from build123d import *

# Parameters (mm, degrees)
SKETCH1_R           = 12.7
BOSS_EXTRUDE1_DEPTH = 7.9248
SKETCH2_R           = 9.525
BOSS_EXTRUDE2_DEPTH = 13.2715
SKETCH3_R           = 5.6388
BOSS_EXTRUDE3_DEPTH = 9.525
BOSS_EXTRUDE4_START = 6.35
SKETCH4_R           = 9.525
BOSS_EXTRUDE4_DEPTH = 6.35
SKETCH5_R           = 8.636
BOSS_EXTRUDE5_DEPTH = 9.525
SKETCH6_R           = 6.35
CUT_EXTRUDE1_DEPTH  = 25.4
SKETCH7_R           = 3.175
CUT_EXTRUDE2_DEPTH  = 32.108519733


with BuildPart() as part:
    # Sketch1 → Boss-Extrude1 (new body)
    with BuildSketch(Plane(origin=(0, 0, 0), x_dir=(0, 0, -1), z_dir=(1, 0, 0))):
        Circle(SKETCH1_R)
    extrude(amount=BOSS_EXTRUDE1_DEPTH)

    # Sketch2 → Boss-Extrude2 (add)
    with BuildSketch(Plane(origin=(7.9248, 0, 0), x_dir=(0, 0, -1), z_dir=(1, 0, 0))):
        Circle(SKETCH2_R)
    extrude(amount=BOSS_EXTRUDE2_DEPTH)

    # Sketch3 → Boss-Extrude3 (add)
    with BuildSketch(Plane(origin=(21.1963, 0, 0), x_dir=(0, 0, -1), z_dir=(1, 0, 0))):
        with Locations(Location((0, 0, 0), (0, 0, 180))):
            Circle(SKETCH3_R)
    extrude(amount=BOSS_EXTRUDE3_DEPTH)

    # Sketch4 → Boss-Extrude4 (add)
    with BuildSketch(Plane.ZY.offset(BOSS_EXTRUDE4_START)):
        with Locations(Location((0, 0, 0), (0, 0, 180))):
            Circle(SKETCH4_R)
    extrude(amount=-BOSS_EXTRUDE4_DEPTH)

    # Sketch5 → Boss-Extrude5 (add)
    with BuildSketch(Plane.ZY.offset(6.35)):
        with Locations(Location((0, 0, 0), (0, 0, 180))):
            Circle(SKETCH5_R)
    extrude(amount=BOSS_EXTRUDE5_DEPTH)

    # Sketch6 → Cut-Extrude1 (cut)
    with BuildSketch(Plane.ZY.offset(15.875)):
        Circle(SKETCH6_R)
    extrude(amount=-CUT_EXTRUDE1_DEPTH, mode=Mode.SUBTRACT)

    # Sketch7 → Cut-Extrude2 (cut, through all)
    with BuildSketch(Plane.ZY.offset(-9.525)):
        Circle(SKETCH7_R)
    extrude(amount=-CUT_EXTRUDE2_DEPTH, mode=Mode.SUBTRACT)


solid = part.part
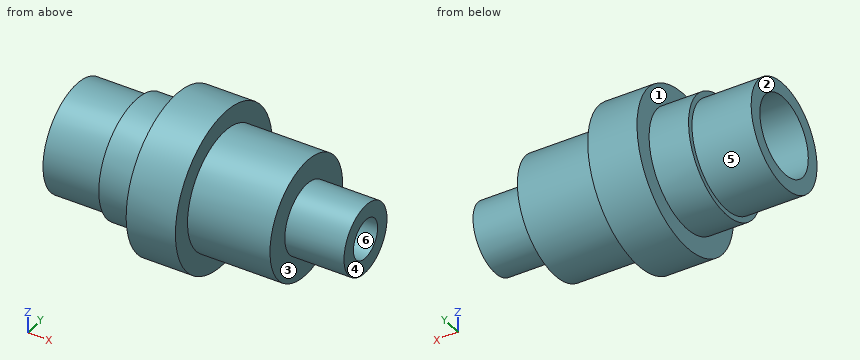
Source: CAD feature listing. Evaluate the final solid. Frame: model axes, mm. Face numbers are marked on the shaded views. A direction names the side the tool comes from. Round coordinates to 2 decimals unless told otherwise and drop trailing zeros. Loops run counter-clockwise (first coordinate to the right, second up) from the corner with the lowest first, then second, coordinate; pieces in that order, holes last. Notation, with made-up numbers: M 14,-15 L 38,-15 A30 cw 38,21 Z; hole C -7,2.25 d2. An arc over 180 degrees is marked long. Return JSON: item names as keys, results as strings. Group by question number.
1. Section query A-A on z = 0. Output: boundary loops of the cut face in (x, y) (3 decimals), and give its area (3 significant figures).
2. Section query C-C on x = 18. Output: boundary loops of the cut face in (y, z) (3 decimals), and give its area (3 significant figures).
3. Mould query, pull axis Z, two halves, no side actions, for the marked faces 4, 5 and 6. Classes: released by +Z, released by -Z, zero draft, split by the parting line, or undercut.
4. Pin query (flat end, axial travel): pin 1 (15 mm diameter, centred on y = 4.5, z = 4.5, fed in from +X); pin 2 (1.5 mm diameter, centred on x = -5.5, z = -8, fed in from -Y); pin 3 (4 mm diameter, centred on y = 6, z = -5, fed in from +X); pin 4 (7.5 mm diameter, centred on y = 0, z = 0, fed in from -X) (3 decimals). Return the tip coordinate at first contact, or that it passes through.
5. Section query D-D on y = 4.5. Output: boundary loops of the cut face in (x, z) (3 decimals).
6. Material intervals for line 1 along Y through (x, z) = (-4.5, 0) (3 decimals); line 2 along Y through (x, z) = (18.5, 0) (3 decimals); line 3 along Z through (x, y) = (-8.5, -0.25), sorted ascending. Write a range as from..to.
7. Reachability of the marked faces 1, 2 and 3 from +Z, -Z, +X, -X, +Y, -Y: full face, straight path, thin tool, end or side. Return the list, or none.
Checks:
{
 "1": {"outline": "M -15.875,-8.636 L -6.35,-8.636 L -6.35,-9.525 L 0,-9.525 L 0,-12.7 L 7.925,-12.7 L 7.925,-9.525 L 21.196,-9.525 L 21.196,-5.639 L 30.721,-5.639 L 30.721,-3.175 L 9.525,-3.175 L 9.525,-6.35 L -15.875,-6.35 Z; M -15.875,6.35 L 9.525,6.35 L 9.525,3.175 L 30.721,3.175 L 30.721,5.639 L 21.196,5.639 L 21.196,9.525 L 7.925,9.525 L 7.925,12.7 L 0,12.7 L 0,9.525 L -6.35,9.525 L -6.35,8.636 L -15.875,8.636 Z", "area": "390 mm²"},
 "2": {"outline": "C 0,0 d19.05; hole C 0,0 d6.35", "area": "253 mm²"},
 "3": {"face 4": "zero draft", "face 5": "split by the parting line", "face 6": "undercut"},
 "4": {"pin 1": "stops at x = 30.72", "pin 2": "stops at y = -6.18", "pin 3": "stops at x = 21.2", "pin 4": "stops at x = 9.525"},
 "5": {"outline": "M -15.875,-7.371 L -6.35,-7.371 L -6.35,-8.395 L 0,-8.395 L 0,-11.876 L 7.925,-11.876 L 7.925,-8.395 L 21.196,-8.395 L 21.196,-3.398 L 30.721,-3.398 L 30.721,3.398 L 21.196,3.398 L 21.196,8.395 L 7.925,8.395 L 7.925,11.876 L 0,11.876 L 0,8.395 L -6.35,8.395 L -6.35,7.371 L -15.875,7.371 L -15.875,4.48 L 9.525,4.48 L 9.525,-4.48 L -15.875,-4.48 Z"},
 "6": {"line 1": "y = -9.525..-6.35, 6.35..9.525", "line 2": "y = -9.525..-3.175, 3.175..9.525", "line 3": "z = -8.63..-6.35, 6.35..8.63"},
 "7": {"face 1": "-X", "face 2": "+Z, -Z, -X, +Y, -Y", "face 3": "+X"}
}
